Part model, mm, in its own coordinate system. A direction names the side the tool comes from. Round coordinates to 2 decimals unless told otherwise and drop trailing zeros. Write each loop counter-clockwise with the first axis right and the second up, starting at its lowest first coordinate (ties: lowest second). Pieces come first, ordered by that corner, then holes.
from build123d import *

# Parameters (mm, degrees)
SKETCH1_W                      = 57
SKETCH1_H                      = 14
BOSS_EXTRUDE1_DEPTH            = 10
CUT_EXTRUDE1_DEPTH             = 3.5
CUT_EXTRUDE2_DEPTH             = 7.5
CBORE_FOR_M3_SHCS1_D           = 3.4
CBORE_FOR_M3_SHCS1_CBORE_D     = 6.5
CBORE_FOR_M3_SHCS1_CBORE_DEPTH = 3
LPATTERN1_COUNT                = 2
LPATTERN1_PITCH                = 45
M3X0_5_TAPPED_HOLE1_D          = 2.5


with BuildPart() as part:
    # Sketch1 → Boss-Extrude1 (new body)
    with BuildSketch(Plane.XY):
        Rectangle(SKETCH1_W, SKETCH1_H)
    extrude(amount=BOSS_EXTRUDE1_DEPTH)

    # Sketch2 → Cut-Extrude1 (cut)
    with BuildSketch(Plane.XY.offset(10)):
        with BuildLine():
            Line((-7, 3), (-7, -3))
            ThreePointArc((-7, -3), (-10, -6), (-13, -3))
            Line((-13, -3), (-13, 3))
            ThreePointArc((-13, 3), (-10, 6), (-7, 3))
        make_face()
        with BuildLine():
            Line((13, 3), (13, -3))
            ThreePointArc((13, -3), (10, -6), (7, -3))
            Line((7, -3), (7, 3))
            ThreePointArc((7, 3), (10, 6), (13, 3))
        make_face()
    extrude(amount=-CUT_EXTRUDE1_DEPTH, mode=Mode.SUBTRACT)

    # Sketch3 → Cut-Extrude2 (cut, through all)
    with BuildSketch(Plane.XY.offset(6.5)):
        with BuildLine():
            Line((-11.75, 3), (-11.75, -3))
            ThreePointArc((-11.75, -3), (-10, -4.75), (-8.25, -3))
            Line((-8.25, -3), (-8.25, 3))
            ThreePointArc((-8.25, 3), (-10, 4.75), (-11.75, 3))
        make_face()
        with BuildLine():
            Line((11.75, -3), (11.75, 3))
            ThreePointArc((11.75, 3), (10, 4.75), (8.25, 3))
            Line((8.25, 3), (8.25, -3))
            ThreePointArc((8.25, -3), (10, -4.75), (11.75, -3))
        make_face()
    extrude(amount=-CUT_EXTRUDE2_DEPTH, mode=Mode.SUBTRACT)

    # CBORE for M3 SHCS1 (through all)
    with Locations(Plane.XY.offset(10)):
        with Locations((-21.910027568, 0)):
            cbore_for_m3_shcs1 = CounterBoreHole(CBORE_FOR_M3_SHCS1_D / 2, CBORE_FOR_M3_SHCS1_CBORE_D / 2, CBORE_FOR_M3_SHCS1_CBORE_DEPTH)

    # LPattern1: CBORE for M3 SHCS1 ×2
    with Locations(*[(i * LPATTERN1_PITCH, 0, 0) for i in range(1, LPATTERN1_COUNT)]):
        add(cbore_for_m3_shcs1, mode=Mode.SUBTRACT)

    # M3x0.5 Tapped Hole1 (through all)
    with Locations(Plane.XY.offset(10)):
        with Locations((0, 0)):
            Hole(M3X0_5_TAPPED_HOLE1_D / 2)


solid = part.part
Q1. Saw through at D-D, the plane y = 0. Give the number of separate pieces and of enclosed holes in the cut face, and give its area (3 significant figures).
Q2. Two-plate mould, pull along X, no slides. Class faces 1 (the flat face through (28.5, 0, 5)), 2 (the flat face through (0, 2, 10)), 3 (the cylindrical face through (-23.53, 0.51, 3.45)): released by +X, released by -X, zero draft, split by the parting line, or undercut.
Q3. Wall check: line 1 (X direction, y = 2.75, z = 1); line 2 (Y direction, x = 23, z = 2.5); line 3 (X direction, y = 0.5, z = 3.25). Give the ranges that are in metal, low to high.
Q4. Tool access for faces 4 (the cylindrical face through (-25.157, 0.143, 8.521)), 5 (the flat face through (-8.25, 0, 3)), 6 (the flat face through (0, 2, 0)): list every direction of +Z, -Z, +X, -X, +Y, -Y with a clear straight run to the whole face (end or side of a thin tool).
Q5. Drop a flat-ended pin along its axis: P1, Ø5.5, axis at x = 23.09, y = 0, coming from the +Z side. Give the stop position or say it passes through.
Q6. Saw through at A-A, the plane x = 0. Write the cut outline in (y, z), and give its area (3 significant figures).
Q7. Saw through at B-B, the plane y = 4.25. Write the cut outline in (x, z), and give its area (3 significant figures).
Q8. Saw through at C-C, the plane z = 2.5. Write the cut outline in (x, y), and give its area (3 significant figures).
Computed:
1. separate pieces: 6
1. enclosed holes: 0
1. area: 371 mm2
2. face 1: released by +X
2. face 2: zero draft
2. face 3: undercut
3. line 1: x = -28.5 to -11.75, -8.25 to 8.25, 11.75 to 28.5
3. line 2: y = -7 to -1.7, 1.7 to 7
3. line 3: x = -28.5 to -23.53, -20.29 to -11.75, -8.25 to -1.15, 1.15 to 8.25, 11.75 to 21.47, 24.71 to 28.5
4. face 4: +Z
4. face 5: +Z, -Z
4. face 6: -Z, +X, -X, +Y, -Y
5. P1: stops at z = 7
6. outline: (-7, 0) - (-1.25, 0) - (-1.25, 10) - (-7, 10) - close; (1.25, 0) - (7, 0) - (7, 10) - (1.25, 10) - close
6. area: 115 mm2
7. outline: (-28.5, 0) - (-11.22, 0) - (-11.22, 6.5) - (-12.73, 6.5) - (-12.73, 10) - (-28.5, 10) - close; (-8.78, 0) - (8.78, 0) - (8.78, 6.5) - (7.27, 6.5) - (7.27, 10) - (-7.27, 10) - (-7.27, 6.5) - (-8.78, 6.5) - close; (11.22, 0) - (28.5, 0) - (28.5, 10) - (12.73, 10) - (12.73, 6.5) - (11.22, 6.5) - close
7. area: 500 mm2
8. outline: (-28.5, -7) - (28.5, -7) - (28.5, 7) - (-28.5, 7) - close; hole circle Ø3.4 at (-21.91, 0); hole (-11.75, -3) arc R1.75 ccw to (-8.25, -3) - (-8.25, 3) arc R1.75 ccw to (-11.75, 3) - close; hole circle Ø2.5 at (0, 0); hole (8.25, -3) arc R1.75 ccw to (11.75, -3) - (11.75, 3) arc R1.75 ccw to (8.25, 3) - close; hole circle Ø3.4 at (23.09, 0)
8. area: 714 mm2
